```python
from build123d import *

# Parameters (mm, degrees)
F1_DEPTH = 15
F2_DEPTH = 8
F4_DEPTH = 15
F5_D     = 9.7
F6_D     = 10
F8_DEPTH = 29.501
F9_R     = 5
F10_R    = 10


with BuildPart() as f1:
    # F0 (on Front) → F1 (new body)
    with BuildSketch(Plane.XZ):
        with BuildLine():
            ThreePointArc((2.8985507246, -19.7888454362), (15.1322670888, -13.0772509632), (20, 0))
            ThreePointArc((20, 0), (15.1322670888, 13.0772509632), (2.8985507246, 19.7888454362))
            ThreePointArc((2.8985507246, 19.7888454362), (-20, 0), (2.8985507246, -19.7888454362))
        make_face()
    extrude(amount=F1_DEPTH)

    # F0 (on Front) → F2 (join)
    with BuildSketch(Plane.XZ):
        with BuildLine():
            ThreePointArc((2.8985507246, 19.7888454362), (15.1322670888, 13.0772509632), (20, 0))
            ThreePointArc((20, 0), (15.1322670888, -13.0772509632), (2.8985507246, -19.7888454362))
            Line((2.8985507246, -19.7888454362), (70.4492753623, -9.8944227181))
            ThreePointArc((70.4492753623, -9.8944227181), (59, 0), (70.4492753623, 9.8944227181))
            Line((70.4492753623, 9.8944227181), (2.8985507246, 19.7888454362))
        make_face()
        with BuildLine():
            ThreePointArc((79, 0), (76.5661335444, 6.5386254816), (70.4492753623, 9.8944227181))
            ThreePointArc((70.4492753623, 9.8944227181), (59, 0), (70.4492753623, -9.8944227181))
            ThreePointArc((70.4492753623, -9.8944227181), (76.5661335444, -6.5386254816), (79, 0))
        make_face()
    extrude(amount=F2_DEPTH)

    # F3 (on Right) → F4 (join, symmetric)
    with BuildSketch(Plane.YZ):
        Polygon((-14.7, 0), (0, 0), (0, 32), (-25.5, 32), (-25.5, 26.0460784735), (-14.7, 17.137655493), align=None)
    extrude(amount=F4_DEPTH, both=True)

    # F5 (through all)
    with Locations(Plane(origin=(0, 0, 0), x_dir=(1, 0, 0), z_dir=(0, 1, 0))):
        with Locations((69, 0)):
            Hole(F5_D / 2)

    # F6 (through all)
    with Locations(Plane(origin=(0, 0, 0), x_dir=(1, 0, 0), z_dir=(0, 1, 0))):
        with Locations((0, 0)):
            Hole(F6_D / 2)

    # F7 (on face) → F8 (cut, through all)
    with BuildSketch(Plane.XY.offset(32)):
        with BuildLine():
            Line((-5, -25.5), (5, -25.5))
            Line((5, -25.5), (4, -20.5))
            ThreePointArc((4, -20.5), (4.7434164903, -19.0811388301), (5, -17.5))
            ThreePointArc((5, -17.5), (0, -12.5), (-5, -17.5))
            ThreePointArc((-5, -17.5), (-4.7434164903, -19.0811388301), (-4, -20.5))
            Line((-4, -20.5), (-5, -25.5))
        make_face()
    extrude(amount=-F8_DEPTH, mode=Mode.SUBTRACT)

    # F9
    f9_edges = [f1.edges().sort_by_distance(p)[0] for p in [
        (15, -12.75, 32),
        (-15, -12.75, 32),
    ]]
    fillet(f9_edges, radius=F9_R)

    # F10
    f10_edges = [f1.edges().sort_by_distance(p)[0] for p in [
        (15, -4, 18.016298),
        (-15, -7.35, 13.228757),
    ]]
    fillet(f10_edges, radius=F10_R)


solid = f1.part
```
The listing builds one solid part. Answer for the finished solid, in the listing's coordinates (mm). A direction names the side the tool comes from. Round coordinates to 2 decimals unless told otherwise and drop trailing zeros. Order: outer loops, then holes, each group sorted by start corner. A loop starts at its lowest first (then second) coordinate and runs counter-clockwise, first axis right, second up. Notation, with made-up numbers: (0.5, -32.5) -> (24.5, -32.5) arc R11 ccw to (24.5, -23.5) -> close; hole circle Ø4 at (8.25, -12). An arc over 180 degrees is marked (long way). Answer as CSV lines item,"result".
Q1. A cutting plane is placed at D-D on z = 1. Determine the outline of the cut face in (x, y).
Computed values:
outline,"(-19.97, -15) -> (-4.9, -15) -> (-4.9, 0) -> (-19.97, 0) -> close; (4.9, -15) -> (19.97, -15) -> (19.97, -8) -> (64.25, -8) -> (64.25, 0) -> (4.9, 0) -> close; (73.75, -8) -> (78.95, -8) -> (78.95, 0) -> (73.75, 0) -> close"
Q2. For a pull along Z with two mould halves and no side action, classify faces 5 (the cylindrical face through (0.651, -7.605, -4.957)), 6 (the flat face through (47.33, -3.94, 13.28)), 7 (the flat face through (10, -25.5, 29)) as +Z half, -Z half, draft (parallel to the pull), parting line (faces both ways), or undercut.
Computed values:
face 5,"undercut"
face 6,"+Z half"
face 7,"draft"
Q3. A cutting plane is placed at C-C on y = -10. Determine the outline of the cut face in (x, z), plus the area to 3 significant figures.
Computed values:
outline,"(-16.67, 11.06) arc R20 ccw (long way) to (15, 13.23) -> (15, 27) arc R5 ccw to (10, 32) -> (-10, 32) arc R5 ccw to (-15, 27) -> (-15, 16.58) arc R10 cw to start; hole circle Ø10 at (0, 0)"
area,"1,590 mm^2"
Q4. Given pin 1 (5 mm diameter, centred on y = -7, z = 22.5, fed in from -X); pin 2 (12 mm diameter, centred on x = 30, z = 19, fed in from -Y); pin 3 (10 mm diameter, centred on y = -3, z = 26.5, fed in from +X), each flat-ended and moving along its own axis, determine where each tip first touches the part or whether it passes through.
Computed values:
pin 1,"stops at x = -15"
pin 2,"stops at y = -8"
pin 3,"stops at x = 16.43"
Q5. Consider line 1 (Z direction, x = 0, y = -5); line 2 (Y direction, x = 9.5, z = 7); line 3 (Z direction, x = 69, y = -2.25). Determine where each line is inside the solid, lowest interval first. Write a range as from..to.
Computed values:
line 1,"z = -20..-5, 5..32"
line 2,"y = -15..0"
line 3,"z = -10.11..-4.85, 4.85..10.11"
Q6. Which of the six approach directions +Z, -Z, +X, -X, +Y, -Y give full straight-line access (tool end or side, diameter ignored) to faces 1 (the flat face through (14, -14.7, 16)), 2 (the flat face through (-14, -14.7, 15)), 3 (the flat face through (-0.3, -15, -5.2)), 4 (the flat face through (4.5, -23, 28.2))?
Computed values:
face 1,"+X, -Y"
face 2,"-X, -Y"
face 3,"-Z, +X, -X, -Y"
face 4,"+Z, -Z, -Y"
Q7. A cutting plane is placed at A-A on y = -3. Determine the outline of the cut face in (x, z), plus the area to 3 significant figures.
Computed values:
outline,"(-16.67, 11.06) arc R20 ccw to (2.9, -19.79) -> (70.45, -9.89) arc R10 ccw to (70.45, 9.89) -> (23.55, 16.76) arc R10 cw to (15, 26.66) -> (15, 27) arc R5 ccw to (10, 32) -> (-10, 32) arc R5 ccw to (-15, 27) -> (-15, 16.58) arc R10 cw to start; hole circle Ø10 at (0, 0); hole circle Ø9.7 at (69, 0)"
area,"3,130 mm^2"
Q8. A cutting plane is placed at B-B on x = 0. Determine the outline of the cut face in (y, z).
Computed values:
outline,"(-15, -20) -> (0, -20) -> (0, -5) -> (-15, -5) -> close; (-12.5, 5) -> (0, 5) -> (0, 32) -> (-12.5, 32) -> close"
